from build123d import *

# Parameters (mm, degrees)
EXTRUDE_1_DEPTH    = 5
SKETCH_3_W         = 20
SKETCH_3_H         = 11
SKETCH_3_H_2       = 7.5
SKETCH_3_H_3       = 15
EXTRUDE_2_DEPTH    = 20
FILLET_1_R         = 5
FILLET_2_R         = 5
HOLE_WIZARD_M3_1_D = 3.6
FILLET_3_R         = 10
HOLE_WIZARD_M3_2_D = 3.6
HOLE_WIZARD_M3_3_D = 3.6
SKETCH_15_W        = 25
SKETCH_15_H        = 15
EXTRUDE_5_DEPTH    = 5
FILLET_8_R         = 5


with BuildPart() as part:
    # 스케치1 → 보스-돌출1 (new body)
    with BuildSketch(Plane(origin=(0, 0, 0), x_dir=(1, 0, 0), z_dir=(0, 1, 0))):
        Polygon((-100, 60), (-70, 60), (-70, 33), (70, 33), (70, 60), (100, 60), (100, -60), (70, -60), (70, -33), (-70, -33), (-70, -60), (-100, -60), align=None)
    extrude(amount=EXTRUDE_1_DEPTH)

    # 스케치3 → 보스-돌출2 (add)
    with BuildSketch(Plane.XZ):
        with Locations((-90, 54.5)):
            Rectangle(SKETCH_3_W, SKETCH_3_H)
        with Locations((-90, 3.75)):
            Rectangle(SKETCH_3_W, SKETCH_3_H_2)
        with Locations((-90, -3.75)):
            Rectangle(SKETCH_3_W, SKETCH_3_H_2)
        with Locations((-90, -54.5)):
            Rectangle(SKETCH_3_W, SKETCH_3_H)
        with Locations((90, 54.5)):
            Rectangle(SKETCH_3_W, SKETCH_3_H)
        with Locations((90, 0)):
            Rectangle(SKETCH_3_W, SKETCH_3_H_3)
        with Locations((90, -54.5)):
            Rectangle(SKETCH_3_W, SKETCH_3_H)
    extrude(amount=EXTRUDE_2_DEPTH)

    # 필렛1
    fillet_1_edges = [part.edges().sort_by_distance(p)[0] for p in [
        (-90, -20, 60),
        (-90, -20, -60),
        (90, -20, 60),
        (90, -20, -60),
    ]]
    fillet(fillet_1_edges, radius=FILLET_1_R)

    # 필렛2
    fillet_2_edges = [part.edges().sort_by_distance(p)[0] for p in [
        (-85, 5, -60),
        (85, 5, -60),
        (85, 5, 60),
        (-85, 5, 60),
    ]]
    fillet(fillet_2_edges, radius=FILLET_2_R)

    # M3 여유 구멍1 (through all)
    with Locations(Plane.ZY.offset(100)):
        with Locations((-3, -5.5), (-3, -14.5), (3.2, -14.5), (3.2, -5.5), (-53.3, -5.5), (-53.3, -14.5), (53.5, -5.5), (53.5, -14.5)):
            Hole(HOLE_WIZARD_M3_1_D / 2)

    # 필렛3
    fillet_3_edges = [part.edges().sort_by_distance(p)[0] for p in [
        (70, 2.5, 33),
        (-70, 2.5, 33),
        (-70, 2.5, -33),
        (70, 2.5, -33),
    ]]
    fillet(fillet_3_edges, radius=FILLET_3_R)

    # M3 여유 구멍2 (through all)
    with Locations(Plane(origin=(0, 5, 0), x_dir=(1, 0, 0), z_dir=(0, 1, 0))):
        with Locations((55.16, 30.5), (19.16, 30.5), (19.16, -30.5), (55.16, -30.5), (57.992156997, -54.362225267)):
            Hole(HOLE_WIZARD_M3_2_D / 2)

    # M3 여유 구멍3 (through all)
    with Locations(Plane(origin=(0, 5, 0), x_dir=(1, 0, 0), z_dir=(0, 1, 0))):
        with Locations((-32.84982536, 9.5), (-2.42900992, -23.37141197), (-7.84982536, 23.5), (-32.84982536, -18.5), (-80, -23.5), (-83.2, 23.5)):
            Hole(HOLE_WIZARD_M3_3_D / 2)

    # 스케치15 → 보스-돌출5 (add)
    with BuildSketch(Plane(origin=(0, 5, 0), x_dir=(1, 0, 0), z_dir=(0, 1, 0))):
        with Locations((13.607404661, -40.5)):
            Rectangle(SKETCH_15_W, SKETCH_15_H)
        with Locations((13.607404661, 40.5)):
            Rectangle(SKETCH_15_W, SKETCH_15_H)
    extrude(amount=-EXTRUDE_5_DEPTH)

    # 필렛8
    fillet_8_edges = [part.edges().sort_by_distance(p)[0] for p in [
        (1.107404661, 2.5, 48),
        (1.107404661, 2.5, 33),
        (26.107404661, 2.5, 33),
        (26.107404661, 2.5, 48),
        (1.107404661, 2.5, -33),
        (1.107404661, 2.5, -48),
        (26.107404661, 2.5, -48),
        (26.107404661, 2.5, -33),
    ]]
    fillet(fillet_8_edges, radius=FILLET_8_R)


solid = part.part
Verification items for the finished model (mm, model axes). A direction names the side the tool comes from. Round coordinates to 2 decimals unless told otherwise and drop trailing zeros. Order: outer loops, then holes, each group sorted by start corner. A loop starts at its lowest first (then second) coordinate and runs counter-clockwise, first axis right, second up. Notation, with made-up numbers: (51, -23.5) -> (110, -23.5) arc R34 cw to (110, 8.5) -> close; hole circle Ø11 at (51.5, 80). An arc over 180 degrees is marked (long way). Put each result on its own line as item: value.
1) Material ranges on line 1 (Y direction, x = -84.25, z = -3); line 2 (X direction, y = 1.5, z = 23.5); line 3 (Z direction, x = 55.16, y = 1.45), recorded low to high.
Final values:
line 1: y = -20 to -16.3, -12.7 to -7.3, -3.7 to 5
line 2: x = -100 to -81.8, -78.2 to -4.22, -0.63 to 100
line 3: z = -33 to -32.3, -28.7 to 28.7, 32.3 to 33
2) Set-up check for faces 5 (the flat face through (-80, -10, 54)), 6 (the flat face through (26.107, 3, 41)), 7 (the flat face through (-90, -10, 49)), 8 (the flat face through (-70, 2, -52)), 9 (the flat face through (-90, -20, -52)): record each of +Z, -Z, +X, -X, +Y, -Y from which the full face is reachable in a straight line by a thin tool's end or side.
Final values:
face 5: +Z, -Z, -Y
face 6: +Z, +Y, -Y
face 7: +X, -X, -Y
face 8: -Z, +Y, -Y
face 9: +Z, -Z, +X, -X, -Y
3) Section check A-A (x = 82). Give the number of separate pieces and of enclosed holes in the cut face, then the cut area to 3 significant figures.
Final values:
separate pieces: 1
enclosed holes: 8
area: 1,240 mm^2
4) Section check C-C (x = 41). Record the cut outline in (y, z).
Final values:
outline: (0, -33) -> (5, -33) -> (5, 33) -> (0, 33) -> close
5) Mould release check, pull along Z, two halves, no side actions. Record for faces 1 (the flat face through (-90, -8, -60)), 2 (the flat face through (-70, 2, 51)), 3 (the cylindrical face through (85, 4, 58)), 4 (the cylindrical face through (-34.513, 2.465, -8.811)): +Z half, -Z half, draft (parallel to the pull), parting line (faces both ways), or undercut.
Final values:
face 1: -Z half
face 2: draft
face 3: +Z half
face 4: undercut
6) Depth check by flat-ended pin: pin 1 (2 mm diameter, centred on y = -14.5, z = 53.5, fed in from +X); pin 2 (4 mm diameter, centred on x = 55.16, z = 30.5, fed in from -Y); pin 3 (6 mm diameter, centred on x = 50, y = -0.5, fed in from +Z); pin 4 (4 mm diameter, centred on y = -14.5, z = 53.5, fed in from +X). Enter the tip coordinate at first touch or a pass-through.
Final values:
pin 1: passes through
pin 2: stops at y = 0
pin 3: stops at z = 33
pin 4: stops at x = 100
